Drawing for the job (mm, zero at the part's lowest x, y, z). A direction names the side the tool comes from. Give positions to 0.01 mm unless a question says otherwise; leave off trailing zeros. Order: outer loops, then holes, each group sorted by start corner. A loop starts at its lowest first (then second) coordinate and runs counter-clockwise, first axis right, second up. Notation, with made-up numbers: (67, 35) -> (119, 35) arc R38 ccw to (119, 74) -> close; hole circle Ø10 at (-2.75, -34). An arc over 180 degrees is marked (long way). Use one line per item in the form item = value. Start each with the question number.
1) Tool access for the marked faces 4 and 5: list every direction of +Z, -Z, +X, -X, +Y, -Y with a clear straight run to the whole face (end or side of a thin tool).
2) Mould opens along X. For the marked faces 1, 2 and 3 say: pulls with the +X half, pulls with the -X half, needs draft (parallel to the pull), parting line crosses it, or undercut.
3) Probe line 1 (Y direction, x = 10, z = 3.25); line 2 (X direction, y = 8.5, z = 1.75); line 3 (Z direction, x = 14.25, y = 6). List the from-to ranges inside material, lowest first.
4) Cut at B-B, the plane y = 24. Give the cut face in (x, z).
5) Cut at A-A, the plane z = 1.15. Give the cut face in (x, y) (1 decimal), and give its area (3 significant figures).
6) Drop a flat-ended pin along its axis: P1, Ø7.5, axis at x = 7.5, y = 19, coming from the -Z side. Give the stop position or say it passes through.
7) Cut at C-C, the plane z = 4.5. Give the cut face in (x, y) (1 decimal).
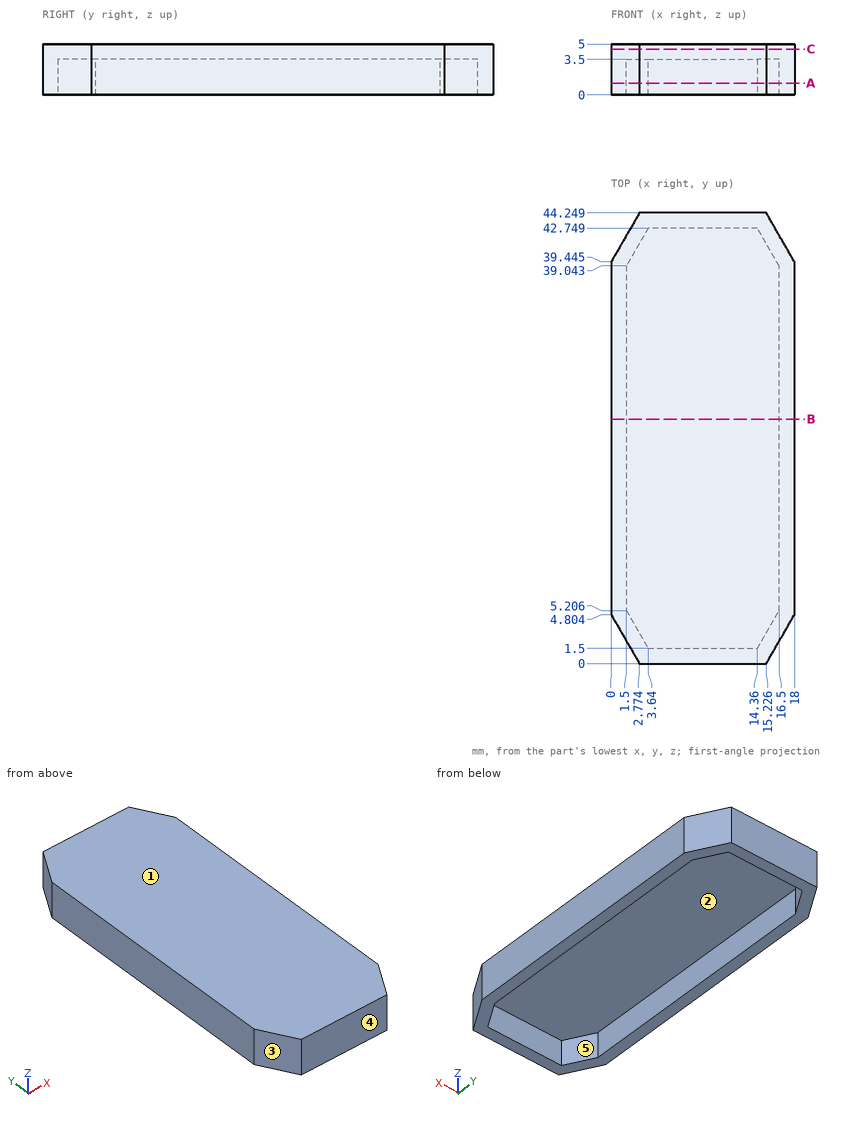
Result:
q1.face_4 = +Z, -Z, +X, -X, -Y
q1.face_5 = -Z
q2.face_1 = needs draft
q2.face_2 = undercut
q2.face_3 = pulls with the -X half
q3.line_1 = 0 to 1.5, 42.75 to 44.25
q3.line_2 = 0 to 1.5, 16.5 to 18
q3.line_3 = 3.5 to 5
q4.outline = (0, 0) -> (1.5, 0) -> (1.5, 3.5) -> (16.5, 3.5) -> (16.5, 0) -> (18, 0) -> (18, 5) -> (0, 5) -> close
q5.outline = (0, 4.8) -> (2.8, 0) -> (15.2, 0) -> (18, 4.8) -> (18, 39.4) -> (15.2, 44.2) -> (2.8, 44.2) -> (0, 39.4) -> close; hole (1.5, 5.2) -> (3.6, 1.5) -> (14.4, 1.5) -> (16.5, 5.2) -> (16.5, 39) -> (14.4, 42.7) -> (3.6, 42.7) -> (1.5, 39) -> close
q5.area = 167 mm²
q6.P1 = 3.5
q7.outline = (0, 4.8) -> (2.8, 0) -> (15.2, 0) -> (18, 4.8) -> (18, 39.4) -> (15.2, 44.2) -> (2.8, 44.2) -> (0, 39.4) -> close
